Work out the finished part from the listing and answer in its coordinate system (mm). A direction names the side the tool comes from. Coordinates: 2 decimals unless noted, no trailing zeros. Write each loop counter-clockwise with the first axis right and the second up, starting at its lowest first coordinate (ties: lowest second). Pieces come first, ordered by that corner, then holes. Notation, with made-up numbers: (48, -39) - (86, -39) arc R16 cw to (86, -12) - close; hole circle Ø7 at (41, 3). An arc over 180 degrees is marked (long way). One line per item, written item: value.
```python
from build123d import *

# Parameters (mm, degrees)
F0_R     = 8.5
F1_DEPTH = 4
F2_R     = 5
F3_DEPTH = 100


with BuildPart() as f1:
    # F0 (on Top) → F1 (new body)
    with BuildSketch(Plane.XY):
        Circle(F0_R)
    extrude(amount=F1_DEPTH)

    # F2 (on Top) → F3 (join)
    with BuildSketch(Plane.XY):
        Circle(F2_R)
    extrude(amount=F3_DEPTH)

    # F4 (on Right) → F5 (revolve)
    with BuildSketch(Plane.YZ):
        with BuildLine():
            Line((0, 104), (0, 100))
            Line((0, 100), (5, 100))
            ThreePointArc((5, 100), (4.472136, 102.236068), (3, 104))
            Line((3, 104), (0, 104))
        make_face()
        with BuildLine():
            ThreePointArc((0, 105), (1.581139, 104.743416), (3, 104))
            ThreePointArc((3, 104), (2.414214, 105.414214), (1, 106))
            Line((1, 106), (0, 106))
            Line((0, 106), (0, 105))
        make_face()
        with BuildLine():
            Line((0, 105), (0, 104))
            Line((0, 104), (3, 104))
            ThreePointArc((3, 104), (1.581139, 104.743416), (0, 105))
        make_face()
    revolve(axis=Axis((0, 0, 103), (0, 0, -1)))


solid = f1.part
```
Item 1: Which of the six approach directions +Z, -Z, +X, -X, +Y, -Y give full straight-line access (tool end or side, diameter ignored) to faces 1 (the face through (-1.08, -4.88, 51.33)), 2 (the face through (0, 0, 0))?
Evaluation:
face 1: +Z
face 2: -Z, +X, -X, +Y, -Y
Item 2: Given pin 1 (3 mm diameter, centred on x = 1, z = 94, fed in from -Y); pin 2 (4 mm diameter, centred on x = 3, z = 83, fed in from +Y); pin 3 (1 mm diameter, centred on y = 2, z = 25.5, fed in from +X), each flat-ended and moving along its own axis, determine where each tip first touches the part or whether it passes through.
Evaluation:
pin 1: stops at y = -5
pin 2: stops at y = 4.9
pin 3: stops at x = 4.77
Item 3: Section C-C, the plane y = 7.25 is taken. Determine the outline of the cut face in (x, z), then the cut area to 3 significant figures.
Evaluation:
outline: (-4.44, 0) - (4.44, 0) - (4.44, 4) - (-4.44, 4) - close
area: 35.5 mm2
Item 4: Section A-A, the plane z = 79 is taken. Determine the outline of the cut face in (x, y), then the cut area to 3 significant figures.
Evaluation:
outline: circle Ø10 at (0, 0)
area: 78.5 mm2
Item 5: Consider probe 1 along Z at (x, y) = (3, -6); probe 2 along Y at (x, z) = (0, 89.5); probe 3 along Z at (x, y) = (-2.75, -0.25). Determine where each line is inside the solid, lowest interval first.
Evaluation:
probe 1: z = 0 to 4
probe 2: y = -5 to 5
probe 3: z = 0 to 104.95
Item 6: Section B-B, the plane x = -6.75 is taken. Determine the outline of the cut face in (y, z), then the cut area to 3 significant figures.
Evaluation:
outline: (-5.17, 0) - (5.17, 0) - (5.17, 4) - (-5.17, 4) - close
area: 41.3 mm2
